Read the model definition and answer for the solid it produces. Units are mm, in the model's axes. A direction names the side the tool comes from. Coordinates: 2 decimals unless noted, no trailing zeros. Loops run counter-clockwise (first coordinate to the right, second up) from the corner with the lowest first, then second, coordinate; pieces in that order, holes last.
from build123d import *

# Parameters (mm, degrees)
SKETCH1_W                  = 1
SKETCH1_H                  = 4
BOSS_EXTRUDE1_DEPTH        = 1
SKETCH3_R                  = 2.95
BOSS_EXTRUDE2_DEPTH        = 54
F_4_1_4_1_DIAMETER_HOLE1_D = 4.1


with BuildPart() as part:
    # Sketch1 → Revolve1 (revolve)
    with BuildSketch(Plane(origin=(0, 0, 0), x_dir=(-1, 0, 0), z_dir=(0, 0, -1))):
        with Locations((-32.5, 2)):
            Rectangle(SKETCH1_W, SKETCH1_H)
    revolve(axis=Axis((33, 0, 0), (-1, 0, 0)))

    # Sketch2 → Boss-Extrude1 (add)
    with BuildSketch(Plane(origin=(0, 0.5, 0), x_dir=(1, 0, 0), z_dir=(0, 1, 0))):
        with BuildLine():
            Line((33, 3.5), (33, -3.5))
            Line((33, -3.5), (40.398405894, -3.5))
            ThreePointArc((40.398405894, -3.5), (43.898405894, 0), (40.398405894, 3.5))
            Line((40.398405894, 3.5), (33, 3.5))
        make_face()
    extrude(amount=-BOSS_EXTRUDE1_DEPTH)

    # Sketch3 → Boss-Extrude2 (add)
    with BuildSketch(Plane.ZY.offset(-32)):
        Circle(SKETCH3_R)
    extrude(amount=BOSS_EXTRUDE2_DEPTH)

    # Ø4.1 (4.1) Diameter Hole1 (through all)
    with Locations(Plane(origin=(0, -0.5, 0), x_dir=(-1, 0, 0), z_dir=(0, -1, 0))):
        with Locations((-40.398405894, 0)):
            Hole(F_4_1_4_1_DIAMETER_HOLE1_D / 2)


solid = part.part
Q1. A cutting plane is placed at B-B (y = -2.25). Give the vertices of the cut face in (x, z).
Findings below:
outline: (-22, -1.91) - (32, -1.91) - (32, -3.31) - (33, -3.31) - (33, 3.31) - (32, 3.31) - (32, 1.91) - (-22, 1.91) - close
Q2. A cutting plane is placed at A-A (z = 1.25). Give the vertices of the cut face in (x, y).
Findings below:
outline: (-22, -2.67) - (32, -2.67) - (32, -3.8) - (33, -3.8) - (33, -0.5) - (38.77, -0.5) - (38.77, 0.5) - (33, 0.5) - (33, 3.8) - (32, 3.8) - (32, 2.67) - (-22, 2.67) - close; (42.02, -0.5) - (43.67, -0.5) - (43.67, 0.5) - (42.02, 0.5) - close
Q3. Straight lines are drawn through the part: probe 1 along Y at (x, z) = (34, 2.5); probe 2 along X at (y, z) = (-3.5, -1.75); probe 3 along X at (y, z) = (-2, 1.5). For each, find the intervals that lie inside material, in ascending order.
Findings below:
probe 1: y = -0.5 to 0.5
probe 2: x = 32 to 33
probe 3: x = -22 to 33
Q4. Determine the mould class of faces 6 (the face through (32, 2, 3)), 7 (the face through (32.493, -0.867, 3.905)), 8 (the face through (38.35, 0.01, -0.09)) for opening direction X: +X half, -X half, draft (parallel to the pull), parting line (faces both ways), or undercut.
Findings below:
face 6: -X half
face 7: draft
face 8: undercut
Q5. Flat-ended cylindrical pins translate along their axes: pin 1 Ø2 at (x, z) = (40.5, 1.5) entering from -Y; pin 2 Ø2 at (x, y) = (20, 2.5) entering from +Z; pin 3 Ø3.5 at (x, z) = (37.5, 1.5) entering from +Y. Find the tip coordinate at first contact, or state that the pin passes through.
Findings below:
pin 1: stops at y = -0.5
pin 2: stops at z = 2.54
pin 3: stops at y = 0.5
Q6. Which of the six approach directions +Z, -Z, +X, -X, +Y, -Y give full straight-line access (tool end or side, diameter ignored) to faces 1 (the face through (5.378, 0.13, -2.947)), 2 (the face through (43.898, 0.007, 0.077)), 3 (the face through (-22, 0, 0)), 4 (the face through (37, 0.5, 0)), 5 (the face through (37, -0.5, 0))?
Findings below:
face 1: -X
face 2: +X, +Y, -Y
face 3: +Z, -Z, -X, +Y, -Y
face 4: +Z, -Z, +X, +Y
face 5: +Z, -Z, +X, -Y
